```python
from build123d import *

# Parameters (mm, degrees)
SZKIC1_R                    = 25
SZKIC1_R_2                  = 22.6
DODANIE_WYCI_GNI_CIE1_DEPTH = 15
SZKIC2_R                    = 1.6
DODANIE_WYCI_GNI_CIE2_DEPTH = 5
ZAOKR_GLENIE3_R             = 2
ZAOKR_GLENIE4_R             = 1
SFAZOWANIE1_SIZE            = 2
SFAZOWANIE1_SIZE2           = 1.154700538


with BuildPart() as part:
    # Szkic1 → Dodanie-wyciągnięcie1 (new body)
    with BuildSketch(Plane.XY):
        Circle(SZKIC1_R)
        Circle(SZKIC1_R_2, mode=Mode.SUBTRACT)
    extrude(amount=DODANIE_WYCI_GNI_CIE1_DEPTH)

    # Szkic2 → Dodanie-wyciągnięcie2 (add)
    with BuildSketch(Plane.XY.offset(15)):
        with BuildLine():
            Line((-22.5, 27.5), (22.5, 27.5))
            ThreePointArc((22.5, 27.5), (26.035533906, 26.035533906), (27.5, 22.5))
            Line((27.5, 22.5), (27.5, -22.5))
            ThreePointArc((27.5, -22.5), (26.035533906, -26.035533906), (22.5, -27.5))
            Line((22.5, -27.5), (-22.5, -27.5))
            ThreePointArc((-22.5, -27.5), (-26.035533906, -26.035533906), (-27.5, -22.5))
            Line((-27.5, -22.5), (-27.5, 22.5))
            ThreePointArc((-27.5, 22.5), (-26.035533906, 26.035533906), (-22.5, 27.5))
        make_face()
        with Locations((-21.213203436, 21.213203436)):
            Circle(SZKIC2_R, mode=Mode.SUBTRACT)
        with Locations((21.213203436, 21.213203436)):
            Circle(SZKIC2_R, mode=Mode.SUBTRACT)
        with Locations((21.213203436, -21.213203436)):
            Circle(SZKIC2_R, mode=Mode.SUBTRACT)
        with Locations((-21.213203436, -21.213203436)):
            Circle(SZKIC2_R, mode=Mode.SUBTRACT)
    extrude(amount=DODANIE_WYCI_GNI_CIE2_DEPTH)

    # Zaokrąglenie3
    zaokr_glenie3_edges = [part.edges().sort_by_distance(p)[0] for p in [
        (-26.035533906, -26.035533906, 15),
        (0, -27.5, 15),
        (26.035533906, -26.035533906, 15),
        (27.5, 0, 15),
        (26.035533906, 26.035533906, 15),
        (0, 27.5, 15),
        (-26.035533906, 26.035533906, 15),
        (-27.5, 0, 15),
    ]]
    fillet(zaokr_glenie3_edges, radius=ZAOKR_GLENIE3_R)

    # Zaokrąglenie4
    zaokr_glenie4_edges = [part.edges().sort_by_distance(p)[0] for p in [
        (-25, 0, 15),
    ]]
    fillet(zaokr_glenie4_edges, radius=ZAOKR_GLENIE4_R)

    # Sfazowanie1
    sfazowanie1_edges = [part.edges().sort_by_distance(p)[0] for p in [
        (-22.6, 0, 0),
    ]]
    sfazowanie1_side = [part.faces().sort_by_distance(p)[0] for p in [
        (-22.6, 0, 7.5),
    ]]
    chamfer(sfazowanie1_edges, length=SFAZOWANIE1_SIZE, length2=SFAZOWANIE1_SIZE2, reference=sfazowanie1_side[0])


solid = part.part
```
Source: CAD feature listing. Evaluate the final solid. Frame: model axes, mm. A direction names the side the tool comes from. Round coordinates to 2 decimals unless told otherwise and drop trailing zeros. Loops run counter-clockwise (first coordinate to the right, second up) from the corner with the lowest first, then second, coordinate; pieces in that order, holes last. Notation, with made-up numbers: M 50,31 L 72,31 A9 ccw 72,43 Z; hole C -3.5,-2.75 d11. An arc over 180 degrees is marked long. Use a Markdown table: item, result. Add a question column.
1. Cut plane A-A, the plane z = 8.25. Output: boundary loops of the cut face in (x, y).
2. Contact query for flat-ended pins moving along their axis: pin 1 (2 mm diameter, centred on x = 20, z = 10, fed in from -Y); pin 2 (3 mm diameter, centred on x = -21.21, y = 21.21, fed in from +Z); pin 3 (4 mm diameter, centred on x = 21.21, y = -21.21, fed in from -Z); pin 4 (3 mm diameter, centred on x = -18.5, z = 12.5, fed in from -Y). Output: stop coordinate, or through.
3. Ray query, line 1 along Y through (x, z) = (0, 10.75); line 2 along X through (y, z) = (-0.5, 3) (3 decimals); line 3 along Z through (x, y) = (3.5, -8). Return the intervals inside material, ascending. Write a range as [from, to].
4. Set-up query: faces 1 (the flat face through (-19, -21, 15)), 2 (the flat face through (-20, 19, 15)), 3 (the cylindrical face through (21.556, 6.788, 8.409)). Return all of +Z, -Z, +X, -X, +Y, -Y with unobstructed straight access to the full face (end or side cutting, diameter ignored); none if empty.
Solution:
| question | item | result |
|---|---|---|
| 1 | outline | C 0,0 d50; hole C 0,0 d45.2 |
| 2 | pin 1 | stops at y = -16.25 |
| 2 | pin 2 | passes through |
| 2 | pin 3 | stops at z = 15 |
| 2 | pin 4 | stops at y = -18.33 |
| 3 | line 1 | y = [-25, -22.6], [22.6, 25] |
| 3 | line 2 | x = [-24.995, -22.594], [22.594, 24.995] |
| 3 | line 3 | z = [15, 20] |
| 4 | face 1 | -Z, -X, -Y |
| 4 | face 2 | -Z, -X, +Y |
| 4 | face 3 | -Z |
